from build123d import *

# Parameters (mm, degrees)
EXTRUDE1_DEPTH     = 12.7
SKETCH5_R          = 3.2639
CUT_EXTRUDE1_DEPTH = 136.152108752
SKETCH6_R          = 4.953
CUT_EXTRUDE2_DEPTH = 131.359174591
SKETCH7_R          = 11.1125
CUT_EXTRUDE3_DEPTH = 131.359174591


with BuildPart() as part:
    # Sketch1 → Extrude1 (new, symmetric)
    with BuildSketch(Plane.XY):
        with BuildLine():
            Line((0, 127), (0, 0))
            Line((0, 0), (-50.8, 0))
            Line((-50.8, 0), (-50.8, 0.254))
            ThreePointArc((-50.8, 0.254), (-49.424543317, 4.111160457), (-45.918869163, 6.227718182))
            Line((-45.918869163, 6.227718182), (-12.70563911, 12.982259955))
            ThreePointArc((-12.70563911, 12.982259955), (-8.140959222, 15.738194493), (-6.35, 20.760538838))
            Line((-6.35, 20.760538838), (-6.35, 120.904))
            ThreePointArc((-6.35, 120.904), (-4.564522938, 125.214522938), (-0.254, 127))
            Line((-0.254, 127), (0, 127))
        make_face()
    extrude(amount=EXTRUDE1_DEPTH, both=True)

    # Sketch5 → Cut-Extrude1 (cut, through all)
    with BuildSketch(Plane.ZY.offset(6.35)):
        with Locations(Location((0, 69.85, 0), (0, 0, 270))):
            Circle(SKETCH5_R)
        with Locations(Location((0, 107.95, 0), (0, 0, 270))):
            Circle(SKETCH5_R)
    extrude(amount=-CUT_EXTRUDE1_DEPTH, mode=Mode.SUBTRACT)

    # Sketch6 → Cut-Extrude2 (cut, through all)
    with BuildSketch(Plane(origin=(0, 7.62, 0), x_dir=(-1, 0, 0), z_dir=(0, 1, 0))):
        with Locations(Location((33.3248, 0, 0), (0, 0, 90))):
            Circle(SKETCH6_R)
    extrude(amount=-CUT_EXTRUDE2_DEPTH, mode=Mode.SUBTRACT)

    # Sketch7 → Cut-Extrude3 (cut, through all)
    with BuildSketch(Plane(origin=(0, 7.62, 0), x_dir=(-1, 0, 0), z_dir=(0, 1, 0))):
        with Locations((33.3248, 0)):
            Circle(SKETCH7_R)
    extrude(amount=CUT_EXTRUDE3_DEPTH, mode=Mode.SUBTRACT)


solid = part.part
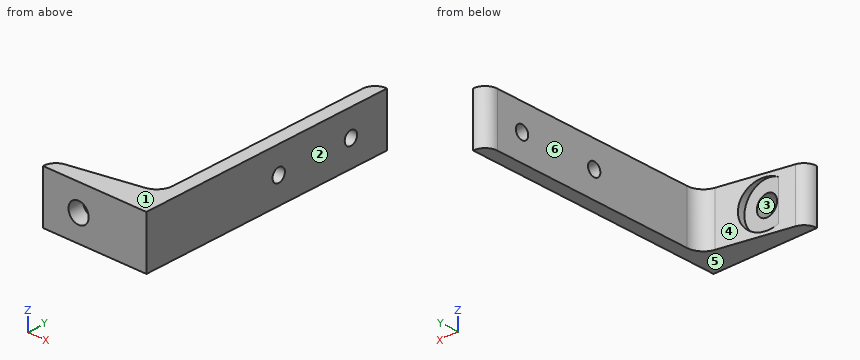
The model under review builds one solid part; all positions refer to its coordinate system, in mm. Face numbers are marked on the shaded views. A direction names the side the tool comes from. Round coordinates to 2 decimals unless told otherwise and drop trailing zeros. Order: outer loops, then holes, each group sorted by start corner. A loop starts at its lowest first (then second) coordinate and runs counter-clockwise, first axis right, second up. Notation, with made-up numbers: (20.5, 69) -> (31.5, 69) arc R8 ccw to (31.5, 78) -> close; hole circle Ø2 at (49, 43.5). An arc over 180 degrees is marked (long way). Return JSON: item names as keys, results as strings.
1. Take a section at B-B (z = 0). State how many separate pieces and enclosed holes the cut face has, then the cut area to 3 significant figures.
Answer block:
{"separate pieces": "4", "enclosed holes": "0", "area": "1,050 mm²"}
2. Insertion check: P1, Ø5, axis at x = -29.5, z = 0.5, coming from the +Y side; P2, Ø5, axis at y = 82, z = 2, coming from the -X side; P3, Ø6, axis at x = -20.5, z = -9.5, coming from the +Y side. Each pin has a flat end and moves straight along its axis. Give the tip position at first contact, or say it passes through.
Answer block:
{"P1": "stops at y = 7.62", "P2": "stops at x = -6.35", "P3": "stops at y = 12.01"}
3. The part is to be moulded in two halves that separate along X. For the marked faces 1, 2, 3 and 4, say which applies: +X half, -X half, draft (parallel to the pull), parting line (faces both ways), or undercut.
Answer block:
{"face 1": "draft", "face 2": "+X half", "face 3": "undercut", "face 4": "-X half"}
4. Take a section at A-A (y = 69.85). Write out the cut boundary in (x, z), then the cut area to 3 significant figures.
Answer block:
{"outline": "(-6.35, -12.7) -> (0, -12.7) -> (0, -3.26) -> (-6.35, -3.26) -> close; (-6.35, 3.26) -> (0, 3.26) -> (0, 12.7) -> (-6.35, 12.7) -> close", "area": "120 mm²"}
5. Take a section at C-C (x = -32). Write out the cut boundary in (y, z).
Answer block:
{"outline": "(0, -12.7) -> (9.06, -12.7) -> (9.06, -11.03) -> (7.62, -11.03) -> (7.62, -4.77) -> (0, -4.77) -> close; (0, 4.77) -> (7.62, 4.77) -> (7.62, 11.03) -> (9.06, 11.03) -> (9.06, 12.7) -> (0, 12.7) -> close"}
6. For the marked faces 5 and 6, list the 3-axis set-ups (+Z, -Z, +X, -X, +Y, -Y) from which the entire face can be reached by the end or side of a thin tool; tool diameter is ignored.
Answer block:
{"face 5": "-Z, +X, -X, +Y, -Y", "face 6": "+Z, -Z, -X, +Y"}
7. For L1, parallel to Z at x = -3.5, y = 107.95; L2, parallel to Y at x = -28, z = 5.5; L3, parallel to X at y = 71.5, z = -9.75, list the stretches that pass through material, from the lowest coordinate up. Write a range as [from, to].
Answer block:
{"L1": "z = [-12.7, -3.26], [3.26, 12.7]", "L2": "y = [0, 7.62]", "L3": "x = [-6.35, 0]"}
